Can you work these out from the model? Positions are in its coordinate system, mm. A direction names the side the tool comes from. Coordinates: 2 decimals unless noted, no trailing zeros. Order: outer loops, then holes, each group sorted by start corner. A loop starts at its lowest first (then second) coordinate and runs counter-clockwise, first axis right, second up. Notation, with made-up numbers: (-4.5, 49.5) -> (-0.5, 49.5) arc R17 ccw to (-0.5, 62.5) -> close; hole circle Ø5 at (86, 55.25). An arc over 180 degrees is marked (long way). Return JSON: item names as keys, results as strings. Group by question number.
1) If we section it at A-A, the plane x = 0: Please give me the cut outline in (y, z) (1 decimal), then the cut area to 3 significant figures.
2) If we section it at C-C, the plane y = -50.8: Please give me the cut outline in (x, z) (3 decimals).
3) For pin 1 (6 mm diameter, centred on x = -1, y = -54.5, fed in from -Z); pin 2 (3 mm diameter, centred on y = -5, z = -0.5, fed in from +X), each with a flat end and sliding along its axis, tell me the tip position at first contact or that it passes through.
4) For faces 1 (the cylindrical face through (-0.34, -1.55, -1.25)), 2 (the flat face through (-7.396, -23.535, 1.565)), which set-ups out of +Z, -Z, +X, -X, +Y, -Y let a thin tool reach every point of the face, with its end or its side?
5) If we section it at B-B, the plane z = -1.9: Please give me the cut outline in (x, y) (1 decimal), then the cut area to 3 significant figures.
6) If I drill on probe 1 along Z at (x, y) = (5.25, -41) (3 decimals); probe 2 along X at (y, z) = (-2.5, 0.8); probe 3 along Y at (x, z) = (-1, -0.5), over which ranges is the centre line in solid material (lowest first)? Write a range as from..to.
7) If we section it at D-D, the plane z = 2.45: Please give me the cut outline in (x, y), then the cut area to 3 significant figures.
from build123d import *

# Parameters (mm, degrees)
F0_R     = 1.5875
F1_DEPTH = 3.175
F2_DEPTH = 2.54


with BuildPart() as f1:
    # F0 (on Top) → F1 (new body)
    with BuildSketch(Plane.XY):
        with BuildLine():
            Line((12.443408, -48.26), (2.488682, 0.508))
            ThreePointArc((2.488682, 0.508), (0, 2.54), (-2.488682, 0.508))
            Line((-2.488682, 0.508), (-12.443408, -48.26))
            ThreePointArc((-12.443408, -48.26), (0, -63.5), (12.443408, -48.26))
        make_face()
        Circle(F0_R, mode=Mode.SUBTRACT)
        Circle(F0_R)
    extrude(amount=F1_DEPTH)

    # F0 (on Top) → F2 (join)
    with BuildSketch(Plane.XY):
        Circle(F0_R)
    extrude(amount=-F2_DEPTH)


solid = f1.part
Result sheet:
{
 "1": {"outline": "(-63.5, 0) -> (-1.6, 0) -> (-1.6, -2.5) -> (1.6, -2.5) -> (1.6, 0) -> (2.5, 0) -> (2.5, 3.2) -> (-63.5, 3.2) -> close", "area": "218 mm2"},
 "2": {"outline": "(-12.7, 0) -> (12.7, 0) -> (12.7, 3.175) -> (-12.7, 3.175) -> close"},
 "3": {"pin 1": "stops at z = 0", "pin 2": "stops at x = 3.9"},
 "4": {"face 1": "-Z", "face 2": "+Z, -Z, -X, +Y"},
 "5": {"outline": "circle Ø3.2 at (0, 0)", "area": "7.92 mm2"},
 "6": {"probe 1": "z = 0..3.175", "probe 2": "x = -3.1..3.1", "probe 3": "y = -1.23..1.23"},
 "7": {"outline": "(-12.44, -48.26) arc R12.7 ccw (long way) to (12.44, -48.26) -> (2.49, 0.51) arc R2.54 ccw to (-2.49, 0.51) -> close", "area": "1,050 mm2"}
}
